from build123d import *
from build123d.topology import SkipClean

# Parameters (mm, degrees)
ESQUISSE1_W                                       = 60.8
ESQUISSE1_H                                       = 121.6
BOSS_EXTRU_1_DEPTH                                = 91.2
ESQUISSE2_W                                       = 60.8
ESQUISSE2_H                                       = 60.8
ENL_V_MAT_EXTRU_1_DEPTH                           = 126.342411019
ESQUISSE3_W                                       = 51.8
ESQUISSE3_H                                       = 51.8
ENL_V_MAT_EXTRU_2_DEPTH                           = 60.8
BOSS_EXTRU_3_DEPTH                                = 4
ESQUISSE6_W                                       = 51.8
ESQUISSE6_H                                       = 51.8
ENL_V_MAT_EXTRU_3_DEPTH                           = 60.8
D_GAGEMENT_1_43_D                                 = 7.14248
FRAISAGE_POUR_VIS_T_TE_FRAIS_E_BOMB_E_D           = 4.3053
FRAISAGE_POUR_VIS_T_TE_FRAIS_E_BOMB_E_DEPTH       = 4.5
FRAISAGE_POUR_VIS_T_TE_FRAIS_E_BOMB_E_CSINK_D     = 7.0866
FRAISAGE_POUR_VIS_T_TE_FRAIS_E_BOMB_E_CSINK_ANGLE = 82
D_GAGEMENT_1_42_D                                 = 7.14248
D_GAGEMENT_1_42_DEPTH                             = 20
BOSS_EXTRU_5_DEPTH                                = 4
CHANFREIN1_SIZE                                   = 4
ESQUISSE26_W                                      = 60.8
ESQUISSE26_H                                      = 182.4
ESQUISSE26_R                                      = 3.57124
BOSS_EXTRU_7_DEPTH                                = 1.35


with BuildPart() as part:
    # Esquisse1 → Boss.-Extru.1 (new, symmetric)
    with BuildSketch(Plane.XY):
        Rectangle(ESQUISSE1_W, ESQUISSE1_H)
    extrude(amount=BOSS_EXTRU_1_DEPTH, both=True)

    # Esquisse2 → Enlèv. mat.-Extru.1 (cut, through all)
    with BuildSketch(Plane.ZY.offset(30.4)):
        with Locations((-60.8, 30.4)):
            Rectangle(ESQUISSE2_W, ESQUISSE2_H)
    enl_v_mat_extru_1 = extrude(amount=-ENL_V_MAT_EXTRU_1_DEPTH, mode=Mode.SUBTRACT)

    # Esquisse3 → Enlèv. mat.-Extru.2 (cut)
    with BuildSketch(Plane(origin=(0, 0, -91.2), x_dir=(-1, 0, 0), z_dir=(0, 0, -1))):
        with Locations((0, -30.4)):
            Rectangle(ESQUISSE3_W, ESQUISSE3_H)
    enl_v_mat_extru_2 = extrude(amount=-ENL_V_MAT_EXTRU_2_DEPTH, mode=Mode.SUBTRACT)

    # Symétrie2: Enlèv. mat.-Extru.1, Enlèv. mat.-Extru.2 across plane
    add(enl_v_mat_extru_1.mirror(Plane.XY), mode=Mode.SUBTRACT)
    add(enl_v_mat_extru_2.mirror(Plane.XY), mode=Mode.SUBTRACT)

    # Esquisse10 → Boss.-Extru.3 (add)
    with BuildSketch(Plane(origin=(27.1, 0, 0), x_dir=(0, 0, -1), z_dir=(1, 0, 0))):
        Polygon((30.4, 60.8), (30.4, 0), (91.2, 0), align=None)
        Polygon((-30.4, 60.8), (-91.2, 0), (-30.4, 0), align=None)
    extrude(amount=-BOSS_EXTRU_3_DEPTH)

    # Esquisse6 → Enlèv. mat.-Extru.3 (cut)
    with BuildSketch(Plane(origin=(0, 60.8, 0), x_dir=(1, 0, 0), z_dir=(0, 1, 0))):
        Rectangle(ESQUISSE6_W, ESQUISSE6_H)
    extrude(amount=-ENL_V_MAT_EXTRU_3_DEPTH, mode=Mode.SUBTRACT)

    # Dégagement 1/43 (through all)
    with Locations(Plane(origin=(27.1, 0, 0), x_dir=(0, 0, -1), z_dir=(1, 0, 0))):
        with Locations((45.6, 15.2), (-45.6, 15.2)):
            Hole(D_GAGEMENT_1_43_D / 2)

    # Fraisage pour vis _ t_te frais_e bomb_e
    with Locations(Plane(origin=(30.4, 0, 0), x_dir=(0, 0, -1), z_dir=(1, 0, 0))):
        with Locations((-60.8, -30.4), (0, 30.4), (60.8, -30.4)):
            CounterSinkHole(FRAISAGE_POUR_VIS_T_TE_FRAIS_E_BOMB_E_D / 2, FRAISAGE_POUR_VIS_T_TE_FRAIS_E_BOMB_E_CSINK_D / 2, depth=FRAISAGE_POUR_VIS_T_TE_FRAIS_E_BOMB_E_DEPTH, counter_sink_angle=FRAISAGE_POUR_VIS_T_TE_FRAIS_E_BOMB_E_CSINK_ANGLE)

    # Dégagement 1/42
    with Locations(Plane(origin=(0, -60.8, 0), x_dir=(-1, 0, 0), z_dir=(0, -1, 0))):
        with Locations((0, 78.7), (0, -78.7)):
            Hole(D_GAGEMENT_1_42_D / 2, depth=D_GAGEMENT_1_42_DEPTH)

    # Esquisse23 → Boss.-Extru.5 (add)
    # profile 1 of 2: a face of its own
    with BuildSketch(Plane.ZY.offset(-23.1)):
        Polygon((-41.197704197, 22.825), (-50.002295803, 22.825), (-54.404591605, 15.2), (-50.002295803, 7.575), (-41.197704197, 7.575), (-36.795408395, 15.2), align=None)
        Polygon((-40.25951001, 15.2), (-42.929755005, 19.825), (-48.270244995, 19.825), (-50.94048999, 15.2), (-48.270244995, 10.575), (-42.929755005, 10.575), align=None, mode=Mode.SUBTRACT)
    # profile 2 of 2: a face of its own
    with BuildSketch(Plane.ZY.offset(-23.1)):
        Polygon((54.404591605, 15.2), (50.002295803, 22.825), (41.197704197, 22.825), (36.795408395, 15.2), (41.197704197, 7.575), (50.002295803, 7.575), align=None)
        Polygon((50.94048999, 15.2), (48.270244995, 19.825), (42.929755005, 19.825), (40.25951001, 15.2), (42.929755005, 10.575), (48.270244995, 10.575), align=None, mode=Mode.SUBTRACT)
    extrude(amount=BOSS_EXTRU_5_DEPTH)

    # Chanfrein1
    chanfrein1_edges = [part.edges().sort_by_distance(p)[0] for p in [
        (23.1, 19.0125, 38.996556296),
        (23.1, 11.3875, 38.996556296),
        (23.1, 7.575, 45.6),
        (23.1, 11.3875, 52.203443704),
        (23.1, 19.0125, 52.203443704),
        (23.1, 22.825, 45.6),
        (23.1, 11.3875, -38.996556296),
        (23.1, 19.0125, -38.996556296),
        (23.1, 7.575, -45.6),
        (23.1, 11.3875, -52.203443704),
        (23.1, 22.825, -45.6),
        (23.1, 19.0125, -52.203443704),
    ]]
    chamfer(chanfrein1_edges, length=CHANFREIN1_SIZE - 0.0001)  # a hair under: the kernel refuses the full size

    # Esquisse26 → Boss.-Extru.7 (add)
    with SkipClean():  # the faces are left unmerged after this step: merging them gives an invalid solid
        with BuildSketch(Plane.XZ.offset(60.8)):
            Rectangle(ESQUISSE26_W, ESQUISSE26_H)
            with Locations(Location((0, 78.7, 0), (0, 0, 270))):
                Circle(ESQUISSE26_R, mode=Mode.SUBTRACT)
            with Locations(Location((0, -78.7, 0), (0, 0, 270))):
                Circle(ESQUISSE26_R, mode=Mode.SUBTRACT)
        extrude(amount=BOSS_EXTRU_7_DEPTH)
    add(part.part.scale(1), mode=Mode.REPLACE)  # the faces are merged on a copy


solid = part.part
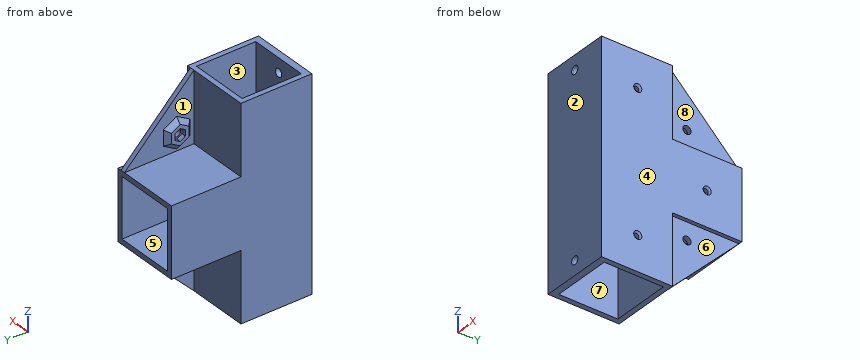
For this review, take the finished solid that the model builds, in its own axes (mm). Face numbers are marked on the shaded views. A direction names the side the tool comes from. Round coordinates to 2 decimals unless told otherwise and drop trailing zeros. Loops run counter-clockwise (first coordinate to the right, second up) from the corner with the lowest first, then second, coordinate; pieces in that order, holes last. Notation, with made-up numbers: (-18, 75.25) - (-3, 75.25) arc R20 cw to (-3, 110.25) - close; hole circle Ø8 at (36, 22). An arc over 180 degrees is marked (long way). One line per item, written item: value. Start each with the question number.
Item 1: Take a section at B-B (z = 0). Give the boundary of the cut face in (x, y), plus the area to 3 significant figures.
Item 2: The part is to be moulded in two halves that separate along Y. For the marked faces 1, 2, 3 and 4, say which applies: +Y half, -Y half, draft (parallel to the pull), parting line (faces both ways), or undercut.
Item 3: Take a section at C-C (y = 53.5). Give the boundary of the cut face in (x, z).
Item 4: Take a section at D-D (x = 13.5). Give the boundary of the cut face in (y, z), plus the area to 3 significant figures.
Item 5: For L1, parallel to Z at x = 27, y = -30; L2, parallel to Z at x = 0, y = -61.9; L3, parallel to Y at x = -8.5, z = -83, list the stretches that pass through material, from the lowest coordinate up.
Item 6: Clearance check with flat-ended pins moving along their axes: pin 1 Ø16 at (x, z) = (-14, -52.5) entering from +Y; pin 2 Ø10 at (y, z) = (16, -43.5) entering from -X; pin 3 Ø3 at (x, z) = (21.5, 45.5) entering from +Y. State where each tip first meets the part, or that it passes through.
Item 7: Take a section at A-A (z = -45.6). State how many separate pieces and enclosed holes the cut face has, plus the area to 3 significant figures.
Item 8: For the marked faces 5, 6, 7 and 8, list the 3-axis set-ups (+Z, -Z, +X, -X, +Y, -Y) from which the entire face can be reached by the end or side of a thin tool; tool diameter is ignored.
Answer below:
1. outline: (-30.4, -62.15) - (30.4, -62.15) - (30.4, 26.86) - (28.8, 28.25) - (25.9, 28.25) - (25.9, 0) - (-25.9, 0) - (-25.9, 60.8) - (-30.4, 60.8) - close; (25.9, 32.55) - (28.8, 32.55) - (30.4, 33.94) - (30.4, 60.8) - (25.9, 60.8) - close
1. area: 4,300 mm2
2. face 1: undercut
2. face 2: -Y half
2. face 3: undercut
2. face 4: draft
3. outline: (-30.4, -30.4) - (23.1, -30.4) - (23.1, -37.7) - (27.1, -37.7) - (27.1, -30.4) - (30.4, -30.4) - (30.4, 30.4) - (27.1, 30.4) - (27.1, 37.7) - (23.1, 37.7) - (23.1, 30.4) - (-30.4, 30.4) - close; hole (-25.9, -25.9) - (25.9, -25.9) - (25.9, 25.9) - (-25.9, 25.9) - close
4. outline: (-62.15, -91.2) - (-56.3, -91.2) - (-56.3, -30.4) - (-4.5, -30.4) - (-4.5, -91.2) - (0, -91.2) - (0, -30.4) - (60.8, -30.4) - (60.8, -25.9) - (0, -25.9) - (0, 25.9) - (60.8, 25.9) - (60.8, 30.4) - (0, 30.4) - (0, 91.2) - (-4.5, 91.2) - (-4.5, 30.4) - (-56.3, 30.4) - (-56.3, 91.2) - (-62.15, 91.2) - close
4. area: 5,580 mm2
5. L1: z = -91.2 to -62.92, -58.68 to 58.68, 62.92 to 91.2
5. L2: z = -91.2 to -82.27, -75.13 to 75.13, 82.27 to 91.2
5. L3: y = -62.15 to -56.3, -4.5 to 0
6. pin 1: stops at y = 0
6. pin 2: stops at x = 19.1
6. pin 3: stops at y = 26.72
7. separate pieces: 2
7. enclosed holes: 1
7. area: 1,290 mm2
8. face 5: +Y
8. face 6: -Z, +X, +Y
8. face 7: -Z
8. face 8: +Z, +X, +Y
